from build123d import *

# Parameters (mm, degrees)
F0_R     = 5
F1_DEPTH = 2.5
F2_SIZE  = 2.49999
F3_DEPTH = 32.5


# Not quite as in the source:
# - a fillet or chamfer is up to 0.001 mm smaller than in the source, because OpenCascade refuses the exact size


with BuildPart() as f1:
    # F0 (on Top) → F1 (new body)
    with BuildSketch(Plane.XY):
        Circle(F0_R)
    extrude(amount=F1_DEPTH)

    # F2 (size 2.5 in the source; OpenCascade refuses exactly that, so slightly less here)
    f2_edges = [f1.edges().sort_by_distance(p)[0] for p in [
        (-5, 0, 2.5),
    ]]
    chamfer(f2_edges, length=F2_SIZE)

    # F3 (add): a face of the model
    f3_faces = [f1.faces().sort_by_distance(p)[0] for p in [
        (0, 0, 2.5),
    ]]
    extrude(f3_faces, amount=F3_DEPTH)


solid = f1.part
Could you check a few things on this model? Use its own coordinates, in mm. A direction names the side the tool comes from. Round coordinates to 2 decimals unless told otherwise and drop trailing zeros. Write each loop counter-clockwise with the first axis right and the second up, starting at its lowest first coordinate (ties: lowest second). Pieces come first, ordered by that corner, then holes. Notation, with made-up numbers: (78.25, -27) - (131.25, -27) arc R8 cw to (131.25, -13) - close; hole circle Ø7 at (-9.75, 27.5). An arc over 180 degrees is marked (long way). Put each result on its own line as item: value. Start each with the question number.
(1) Will these pins go through, and if not, where does the flat tip stop? pin 1 (6 mm diameter, centred on y = -3.5, z = 27, fed in from -X); pin 2 (5 mm diameter, centred on x = -2, z = 26, fed in from -Y); pin 3 (1 mm diameter, centred on x = -3.5, z = 12.5, fed in from -Y); pin 4 (6 mm diameter, centred on y = -2, z = 24.5, fed in from +X).
(2) I want a section at C-C, the plane z = 18.5. Please give me the cut outline in (x, y).
(3) For faces 1 (the flat face through (0, 0, 35)), 2 (the cylindrical face through (-0.54, -2.44, 18.52)), which set-ups out of +Z, -Z, +X, -X, +Y, -Y let a thin tool reach every point of the face, with its end or its side?
(4) I need wall thicknesses on probe 1 along Y at (x, z) = (0, 32); probe 2 along X at (y, z) = (0, 2); probe 3 along Z at (x, y) = (3.25, 3.5). Which ranges of each line are inside material? Lowest first, please.
Here are the results:
1. pin 1: stops at x = -2.45
1. pin 2: stops at y = -2.5
1. pin 3: passes through
1. pin 4: stops at x = 2.5
2. outline: circle Ø5 at (0, 0)
3. face 1: +Z, +X, -X, +Y, -Y
3. face 2: +Z
4. probe 1: y = -2.5 to 2.5
4. probe 2: x = -3 to 3
4. probe 3: z = 0 to 0.22
